Autodesk Inventor part; units mm, degrees
ref_plane "YZ Plane" through (0, 0, 0) normal (1, 0, 0) x (0, 1, 0)
ref_plane "XZ Plane" through (0, 0, 0) normal (0, 1, 0) x (-1, 0, 0)
ref_plane "XY Plane" through (0, 0, 0) normal (0, 0, 1) x (1, 0, 0)
sketch "Sketch1" plane through (0, 0, 0) normal (0, 1, 0) x (-1, 0, 0)
  line L0 (-125, -125) -> (125, -125)
  line L1 (125, -125) -> (125, 125)
  line L2 (125, 125) -> (-125, 125)
  line L3 (-125, 125) -> (-125, -125)
  line L4 (-125, -125) -> (125, 125) construction
  line L5 (125, -125) -> (-125, 125) construction
  point P0 (0, 0)
  dimension "Width" = 250
  dimension "Length" = 250
extrude "Main Body Extrusion" add sketch "Sketch1" along normal blind 4
sketch "Sketch3" plane through (0, 4, 0) normal (0, 1, 0) x (1, 0, 0)
  line L0 (96, -96) -> (-96, -96)
  line L1 (-96, -96) -> (-96, 96)
  line L2 (-96, 96) -> (96, 96)
  line L3 (96, -96) -> (-96, 96) construction
  line L4 (-96, -96) -> (96, 96) construction
  line L5 (-125, 125) -> (-125, -125)
  line L6 (125, -125) -> (125, 125)
  line L7 (-125, -125) -> (125, -125)
  line L8 (100, -100) -> (-100, -100)
  line L9 (-100, -100) -> (-100, 100)
  line L10 (-100, 100) -> (100, 100)
  line L11 (100, -100) -> (-100, 100) construction
  line L12 (-100, -100) -> (100, 100) construction
  line L13 (96, 96) -> (100, 96)
  line L14 (96, -96) -> (100, -96)
  line L15 (100, 100) -> (100, 96)
  line L16 (100, -96) -> (100, -100)
  point P0 (0, 0)
  dimension "d16" = 192
  dimension "d17" = 200
  dimension "d18" = 200
extrude "Extrusion3" add sketch "Sketch3" along normal blind 50 from surface at 0
sketch "Sketch8" plane through (0, 4, 0) normal (0, 1, 0) x (1, 0, 0)
  line L0 (100, 100) -> (100, 96)
  line L1 (-96, 96) -> (-96, -96)
  line L2 (100, 96) -> (-96, 96)
  line L3 (-125, -125) -> (125, -125)
  line L4 (89, 96) -> (93, 96)
  line L5 (93, 96) -> (93, -125)
  line L6 (93, -125) -> (89, -125)
  line L7 (89, -125) -> (89, 96)
  line L8 (89, -96) -> (85, -96)
  line L9 (85, -96) -> (85, 96)
  line L10 (85, 96) -> (89, 96)
  line L11 (89, 96) -> (89, -96)
  line L12 (93, 96) -> (97, 96)
  line L13 (97, 96) -> (97, -96)
  line L14 (97, -96) -> (93, -96)
  line L15 (93, -96) -> (93, 96)
  point P0 (0, 0)
  point P1 (89, -125)
  dimension "d39" = 4
  dimension "d40" = 185
  dimension "d47" = 4
  dimension "d48" = 4
extrude "Extrusion8" cut sketch "Sketch8" along normal blind 2 contours L13 L14 L5 L2 | L7 L8 L9 L2
sketch "Sketch9" plane through (-100, 54, 100) normal (0, 0, 1) x (1, 0, 0)
  line L0 (0, -50) -> (200, -50)
  line L1 (193.0019, -50) -> (189.0019, -50)
  line L2 (189.0019, -50) -> (189.0019, -5)
  line L3 (189.0019, -5) -> (193.0019, -5)
  line L4 (193.0019, -5) -> (193.0019, -50)
  point P0 (100, -54)
  dimension "d41" = 4
  dimension "d42" = 45
extrude "Extrusion9" cut sketch "Sketch9" against normal up to surface (4 mm away)
sketch "Sketch10" plane through (-100, 54, -100) normal (0, 1, 0) x (1, 0, 0)
  line L0 (0, -200) -> (0, 0)
  line L1 (200, 0) -> (200, -4)
  line L2 (0, -200) -> (200, -200)
  line L3 (200, -200) -> (200, 0)
  line L4 (200, 0) -> (0, 0)
  line L5 (0, 0) -> (0, -200)
  point P0 (100, -100)
extrude "Extrusion10" add sketch "Sketch10" along normal blind 4
sketch "Sketch11" plane through (-100, 58, -100) normal (0, 1, 0) x (1, 0, 0)
  line L0 (50, -150) -> (150, -150)
  line L1 (150, -150) -> (150, -50)
  line L2 (150, -50) -> (50, -50)
  line L3 (50, -50) -> (50, -150)
  line L4 (50, -150) -> (150, -50) construction
  line L5 (150, -150) -> (50, -50) construction
  point P0 (100, -100)
  point P1 (62.5, -62.5)
  point P2 (62.5, -137.5)
  point P3 (137.5, -137.5)
  point P4 (137.5, -62.5)
  dimension "d56" = 100
  dimension "d57" = 100
  dimension "d58" = 12.5
  dimension "d59" = 12.5
  dimension "d62" = 360
hole "Hole1" at (-37.5, 58, -37.5) at (37.5, 58, -37.5) at (37.5, 58, 37.5) at (-37.5, 58, 37.5) direction (0, -1, 0) diameter 5 depth 4
properties part number "Acrylic Casing" material "Acetal Resin, White"
Verification items for the finished model (mm, model axes). A direction names the side the tool comes from. Coordinates: 2 decimals unless noted, no trailing zeros. Write each loop counter-clockwise with the first axis right and the second up, starting at its lowest first coordinate (ties: lowest second). Pieces come first, ordered by that corner, then holes. Notation, with made-up numbers: (-10.5, 78.5) -> (27.5, 78.5) arc R10 cw to (27.5, 97.5) -> close; hole circle Ø1 at (23.5, -2.75). An arc over 180 degrees is marked (long way). One line per item, written item: value. Start each with the question number.
Q1. Cross-section at D-D on x = 103. Enter the section's corners in (y, z), and give its area (3 significant figures).
Q2. Thickness scan on L1, parallel to X at y = 55, z = 37; L2, parallel to X at y = 56.15, z = -37.5. Record the ranges inside material, lowest first. Write a range as from..to.
Q3. Go/stop test with flat-tipped pins: P1, Ø6, axis at x = 37.5, z = -37.5, coming from the +Y side; P2, Ø12, axis at x = 1, y = 49.5, coming from the -Z side; P3, Ø2, axis at y = 21.5, z = 98.5, coming from the -X side; P4, Ø10, axis at x = 87.5, y = 36, coming from the +Z side. Record where each tip stops, or that it passes through.
Q4. Cross-section at B-B on x = -11. Enter the section's corners in (y, z).
Q5. Access from +Z, -Z, +X, -X, +Y, -Y to the whole of each face (thin tool, end or side, straight path). Record for faces 4 (the flat face through (100, 55, 30)), 5 (the flat face through (-1, 31, 100)), 6 (the flat face through (1, 31, -100)), 7 (the flat face through (1, 54, -1)).
Q6. Mould release check, pull along Y, two halves, no side actions. Record for faces 1 (the flat face through (2, 0, 2)), 2 (the flat face through (-100, 31, 1)), 3 (the flat face through (-96, 29, 1)): pulls with the +Y half, pulls with the -Y half, needs draft (parallel to the pull), parting line crosses it, or undercut.
Q7. Cross-section at C-C on z = 24. Enter the section's corners in (x, y).
Q8. Cross-section at A-A on y = 27. Enter the section's corners in (x, z).
Checked values:
1. outline: (0, -125) -> (4, -125) -> (4, 125) -> (0, 125) -> close
1. area: 1,000 mm²
2. L1: x = -100..-39.95, -35.05..35.05, 39.95..100
2. L2: x = -100..-40, -35..35, 40..100
3. P1: stops at y = 58
3. P2: stops at z = -100
3. P3: stops at x = -100
3. P4: stops at z = 100
4. outline: (0, -125) -> (4, -125) -> (4, -100) -> (58, -100) -> (58, 100) -> (4, 100) -> (4, 125) -> (0, 125) -> close; hole (4, -96) -> (54, -96) -> (54, 96) -> (4, 96) -> close
5. face 4: +Z, -Z, +X, +Y
5. face 5: +Z, +X, -X, +Y
5. face 6: -Z, +X, -X, +Y
5. face 7: +X
6. face 1: pulls with the -Y half
6. face 2: needs draft
6. face 3: undercut
7. outline: (-125, 0) -> (125, 0) -> (125, 4) -> (-96, 4) -> (-96, 54) -> (100, 54) -> (100, 58) -> (-100, 58) -> (-100, 4) -> (-125, 4) -> close
8. outline: (-100, -100) -> (100, -100) -> (100, -96) -> (-96, -96) -> (-96, 96) -> (89, 96) -> (89, 100) -> (-100, 100) -> close; (93, 96) -> (100, 96) -> (100, 100) -> (93, 100) -> close
